from build123d import *

# Parameters (mm, degrees)
SKETCH1_W           = 177.8
SKETCH1_H           = 63.5
BOSS_EXTRUDE1_DEPTH = 3.175
SKETCH3_W           = 3.175
SKETCH3_H           = 63.5
BOSS_EXTRUDE2_DEPTH = 38.1
SKETCH4_W           = 63.5
SKETCH4_H           = 3.175
BOSS_EXTRUDE3_DEPTH = 12.7
SKETCH5_R           = 2.54
CUT_EXTRUDE1_DEPTH  = 12.7
BOSS_EXTRUDE4_DEPTH = 63.5


with BuildPart() as part:
    # Sketch1 → Boss-Extrude1 (new body)
    with BuildSketch(Plane(origin=(0, 0, 0), x_dir=(1, 0, 0), z_dir=(0, 1, 0))):
        Rectangle(SKETCH1_W, SKETCH1_H)
    extrude(amount=BOSS_EXTRUDE1_DEPTH)

    # Sketch3 → Boss-Extrude2 (add)
    with BuildSketch(Plane(origin=(0, 3.175, 0), x_dir=(1, 0, 0), z_dir=(0, 1, 0))):
        with Locations((-90.4875, 0)):
            Rectangle(SKETCH3_W, SKETCH3_H)
        with Locations((90.4875, 0)):
            Rectangle(SKETCH3_W, SKETCH3_H)
    extrude(amount=-BOSS_EXTRUDE2_DEPTH)

    # Sketch4 → Boss-Extrude3 (add)
    with BuildSketch(Plane(origin=(92.075, 0, 0), x_dir=(0, 0, -1), z_dir=(1, 0, 0))):
        with Locations((0, -33.3375)):
            Rectangle(SKETCH4_W, SKETCH4_H)
    boss_extrude3 = extrude(amount=BOSS_EXTRUDE3_DEPTH)

    # Sketch5 → Cut-Extrude1 (cut)
    with BuildSketch(Plane.XZ.offset(34.925)):
        with Locations(Location((95.25, -15.24, 0), (0, 0, 270))):
            Circle(SKETCH5_R)
    cut_extrude1 = extrude(amount=-CUT_EXTRUDE1_DEPTH, mode=Mode.SUBTRACT)

    # Mirror1: Boss-Extrude3, Cut-Extrude1 across plane
    add(boss_extrude3.mirror(Plane(origin=(0, 0, 0), x_dir=(0, 0, 1), z_dir=(1, 0, 0))))
    add(cut_extrude1.mirror(Plane(origin=(0, 0, 0), x_dir=(0, 0, 1), z_dir=(1, 0, 0))), mode=Mode.SUBTRACT)

    # Sketch6 → Boss-Extrude4 (add)
    with BuildSketch(Plane.XY.offset(31.75)):
        Polygon((58.674, 0), (58.674, -11.43), (66.294, -11.43), (66.294, -8.89), (62.484, -8.89), (62.484, 0), align=None)
        Polygon((82.55, 0), (82.55, -11.43), (74.93, -11.43), (74.93, -8.89), (78.74, -8.89), (78.74, 0), align=None)
    extrude(amount=-BOSS_EXTRUDE4_DEPTH)


solid = part.part
Model file for the job. Use its own axes, mm. A direction names the side the tool comes from. Give positions to 0.01 mm unless a question says otherwise; leave off trailing zeros. Order: outer loops, then holes, each group sorted by start corner. A loop starts at its lowest first (then second) coordinate and runs counter-clockwise, first axis right, second up. Notation, with made-up numbers: M 47.25,-6 L 100.25,-6 A34 cw 100.25,29 Z; hole C 64.5,-2 d10. An arc over 180 degrees is marked long. Put each result on its own line as item: value. Start each with the question number.
(1) Pin check, flat tips, straight feed: pin 1 Ø1.5 at (y, z) = (-30.5, 3) entering from -X (3 decimals); pin 2 Ø3 at (x, z) = (-95.25, -15.24) entering from +Y; pin 3 Ø17.5 at (y, z) = (-15.5, 2.5) entering from +X (3 decimals); pin 4 Ø3 at (x, z) = (85, -7) entering from -Y. Stop position of each tip, or through.
(2) Tool access for faces 1 (the face through (77, -8.89, 0)), 2 (the face through (92.075, -14, 0)), 3 (the face through (79, -11.43, 0)), 4 (the face through (-92.075, -14, 0)): list every direction of +Z, -Z, +X, -X, +Y, -Y with a clear straight run to the whole face (end or side of a thin tool).
(3) Band-saw the part on D-D on z = -5. Give the cut face in (x, y) (3 decimals).
(4) Band-saw the part on A-A on z = -15.24. Count the separate pieces of the cut face and the enclosed holes in it, then the cut area to 3 significant figures.
(5) Band-saw the part on C-C on x = -95.25. Give the cut face in (y, z) (3 decimals), then the cut area to 3 significant figures.
(6) Band-saw the part on B-B on y = -26.5. Give the cut face in (x, z) (3 decimals), then the cut area to 3 significant figures.
(7) Drill centre lines: L1, parallel to X at y = -4.5, z = -14 (3 decimals); L2, parallel to X at y = -11, z = 21.5 (3 decimals); L3, parallel to X at y = -28, z = -12 (3 decimals). Where is each one in solid material? Low to high. Write a range as [from, to].
(8) Pull direction Z, two halves, no side cores. Call faces 5 (the face through (97.77, -33.36, -14.91)), 6 (the face through (62.484, -5, 0)), 7 (the face through (8, 1, -31.75)), 8 (the face through (-97.77, -33.36, -14.91)): released by +Z, released by -Z, zero draft, split by the parting line, or undercut.
Results below:
1. pin 1: stops at x = -92.075
1. pin 2: passes through
1. pin 3: stops at x = 92.075
1. pin 4: stops at y = 0
2. face 1: +Z, -Z
2. face 2: +Z, -Z, +X, +Y
2. face 3: +Z, -Z, -Y
2. face 4: +Z, -Z, -X, +Y
3. outline: M -104.775,-34.925 L -88.9,-34.925 L -88.9,0 L 58.674,0 L 58.674,-11.43 L 66.294,-11.43 L 66.294,-8.89 L 62.484,-8.89 L 62.484,0 L 78.74,0 L 78.74,-8.89 L 74.93,-8.89 L 74.93,-11.43 L 82.55,-11.43 L 82.55,0 L 88.9,0 L 88.9,-34.925 L 104.775,-34.925 L 104.775,-31.75 L 92.075,-31.75 L 92.075,3.175 L -92.075,3.175 L -92.075,-31.75 L -104.775,-31.75 Z
4. separate pieces: 3
4. enclosed holes: 0
4. area: 961 mm2
5. outline: M -34.925,-31.75 L -31.75,-31.75 L -31.75,-17.78 L -34.925,-17.78 Z; M -34.925,-12.7 L -31.75,-12.7 L -31.75,31.75 L -34.925,31.75 Z
5. area: 185 mm2
6. outline: M -92.075,-31.75 L -88.9,-31.75 L -88.9,31.75 L -92.075,31.75 Z; M 88.9,-31.75 L 92.075,-31.75 L 92.075,31.75 L 88.9,31.75 Z
6. area: 403 mm2
7. L1: x = [-92.075, -88.9], [58.674, 62.484], [78.74, 82.55], [88.9, 92.075]
7. L2: x = [-92.075, -88.9], [58.674, 66.294], [74.93, 82.55], [88.9, 92.075]
7. L3: x = [-92.075, -88.9], [88.9, 92.075]
8. face 5: undercut
8. face 6: zero draft
8. face 7: released by -Z
8. face 8: undercut
